Design review of the part built by this model. Coordinates are the model's own, in mm. A direction names the side the tool comes from. Coordinates: 2 decimals unless noted, no trailing zeros. Loops run counter-clockwise (first coordinate to the right, second up) from the corner with the lowest first, then second, coordinate; pieces in that order, holes last. Notation, with made-up numbers: (86.25, -40) - (126.25, -40) arc R26 cw to (126.25, -10) - close; hole circle Ø2 at (83, 58). An arc over 180 degrees is marked (long way). Answer in a Markdown table with one row per item. Add a question column.
(1) To check wall thickness, follow L1, parallel to Y at x = 0, z = 3.9; L2, parallel to X at y = 13, z = 17.5; L3, parallel to X at y = -52, z = 24.5. State the ranges of each line that lie inside material, in increasing order. Write a range as [from, to].
(2) The part is to be moulded in two halves that separate along X. For faces 1 (the face through (77.35, -77.61, 2.46)), 2 (the face through (-109.99, -1.47, 2.46)), 3 (the face through (-20.765, -39.923, 92.605)), 4 (the face through (-66, -73, 5)), say which applies: released by +X, released by -X, zero draft, split by the parting line, or undercut.
(3) For faces 5 (the face through (-41, 19, 100)), 6 (the face through (-47.69, 15.02, 92.4)), list the 3-axis set-ups (+Z, -Z, +X, -X, +Y, -Y) from which the entire face can be reached by the end or side of a thin tool; tool diameter is ignored.
(4) We need section A-A, the plane y = 0. Write out the cut boundary in (x, z).
(5) We need section D-D, the plane z = 32.5. Write out the cut boundary in (x, y).
(6) Clearance check with flat-ended pins moving along their axes: pin 1 (12 mm diameter, centred on y = -21, z = 70, fed in from -X); pin 2 (1 mm diameter, centred on y = -5, z = 15, fed in from -X); pin 3 (7 mm diameter, centred on x = 79.73, y = 75.78, fed in from +Z). State where each tip first meets the part, or that it passes through.
(7) We need section C-C, the plane z = 13. Write out the cut boundary in (x, y), plus the area to 3 significant figures.
from build123d import *

# Parameters (mm, degrees)
F0_R     = 3
F0_R_2   = 95
F3_DEPTH = 5


with BuildPart() as f2:
    # F1 (on Front) → F2 (revolve)
    with BuildSketch(Plane.XZ):
        Polygon((-98, 5), (-98, 0), (-93, 0), (-93, 5), (-45, 85), (-45, 100), (-50, 100), (-50, 85), align=None)
    revolve(axis=Axis((0, 0, 50), (0, 0, -1)))

    # F0 (on Top) → F3 (join)
    with BuildSketch(Plane.XY):
        with BuildLine():
            Line((-89.325313, 78.598246), (-102.908732, 38.856053))
            Line((-102.908732, 38.856053), (-105.163031, 32.260454))
            ThreePointArc((-105.163031, 32.260454), (-109.982614, -1.955642), (-103.949644, -35.978765))
            Line((-103.949644, -35.978765), (-89.583886, -77.484232))
            ThreePointArc((-89.583886, -77.484232), (-86.476317, -83.165038), (-80.539903, -85.751064))
            Line((-80.539903, -85.751064), (-41.985508, -101.672106))
            ThreePointArc((-41.985508, -101.672106), (-0.564426, -109.998552), (40.939922, -102.097614))
            Line((40.939922, -102.097614), (82.964931, -85.246088))
            ThreePointArc((82.964931, -85.246088), (87.066641, -82.578532), (89.411846, -78.284362))
            Line((89.411846, -78.284362), (104.028902, -35.74895))
            ThreePointArc((104.028902, -35.74895), (109.999998, -0.018173), (104.040709, 35.714576))
            Line((104.040709, 35.714576), (89.353771, 78.499332))
            Line((89.353771, 78.499332), (88.99239, 79.552075))
            ThreePointArc((88.99239, 79.552075), (86.831614, 82.823834), (83.579002, 85.013326))
            Line((83.579002, 85.013326), (83.317816, 85.117976))
            Line((83.317816, 85.117976), (40.912133, 102.108752))
            ThreePointArc((40.912133, 102.108752), (-0.081717, 109.99997), (-41.063798, 102.047854))
            Line((-41.063798, 102.047854), (-82.349187, 85.434718))
            ThreePointArc((-82.349187, 85.434718), (-86.72871, 82.926152), (-89.325313, 78.598246))
        make_face()
        with Locations((-79.729493, -75.783956)):
            Circle(F0_R, mode=Mode.SUBTRACT)
        with Locations((79.729493, -75.783956)):
            Circle(F0_R, mode=Mode.SUBTRACT)
        with Locations((-79.729493, 75.783956)):
            Circle(F0_R, mode=Mode.SUBTRACT)
        Circle(F0_R_2, mode=Mode.SUBTRACT)
        with Locations((79.729493, 75.783956)):
            Circle(F0_R, mode=Mode.SUBTRACT)
    extrude(amount=F3_DEPTH)


solid = f2.part
Responses:
| question | item | result |
|---|---|---|
| 1 | L1 | y = [-110, -93], [93, 110] |
| 1 | L2 | x = [-89.56, -84.51], [84.51, 89.56] |
| 1 | L3 | x = [-68.87, -62.5], [62.5, 68.87] |
| 2 | face 1 | undercut |
| 2 | face 2 | released by -X |
| 2 | face 3 | undercut |
| 2 | face 4 | zero draft |
| 3 | face 5 | +Z, +X, -X, +Y, -Y |
| 3 | face 6 | +Z |
| 4 | outline | (-110, 0) - (-93, 0) - (-93, 5) - (-45, 85) - (-45, 100) - (-50, 100) - (-50, 85) - (-98, 5) - (-110, 5) - close; (45, 85) - (93, 5) - (93, 0) - (110, 0) - (110, 5) - (98, 5) - (50, 85) - (50, 100) - (45, 100) - close |
| 5 | outline | circle Ø163 at (0, 0); hole circle Ø153 at (0, 0) |
| 6 | pin 1 | stops at x = -59.46 |
| 6 | pin 2 | stops at x = -92.17 |
| 6 | pin 3 | stops at z = 5 |
| 7 | outline | circle Ø186.4 at (0, 0); hole circle Ø176.4 at (0, 0) |
| 7 | area | 2,850 mm2 |
